Check sheet for the drawn part. Datum: minimum x, y, z corner. Units: mm. A direction names the side the tool comes from. Round coordinates to 2 decimals unless told otherwise and drop trailing zeros. Order: outer loops, then holes, each group sorted by start corner. A loop starts at its lowest first (then second) coordinate and runs counter-clockwise, first axis right, second up. Notation, with made-up numbers: (37.5, 68) -> (68.5, 68) arc R25 ccw to (68.5, 91) -> close; hole circle Ø6 at (-14.5, 69). An arc over 180 degrees is marked (long way). Answer in a Markdown table with one row per item.
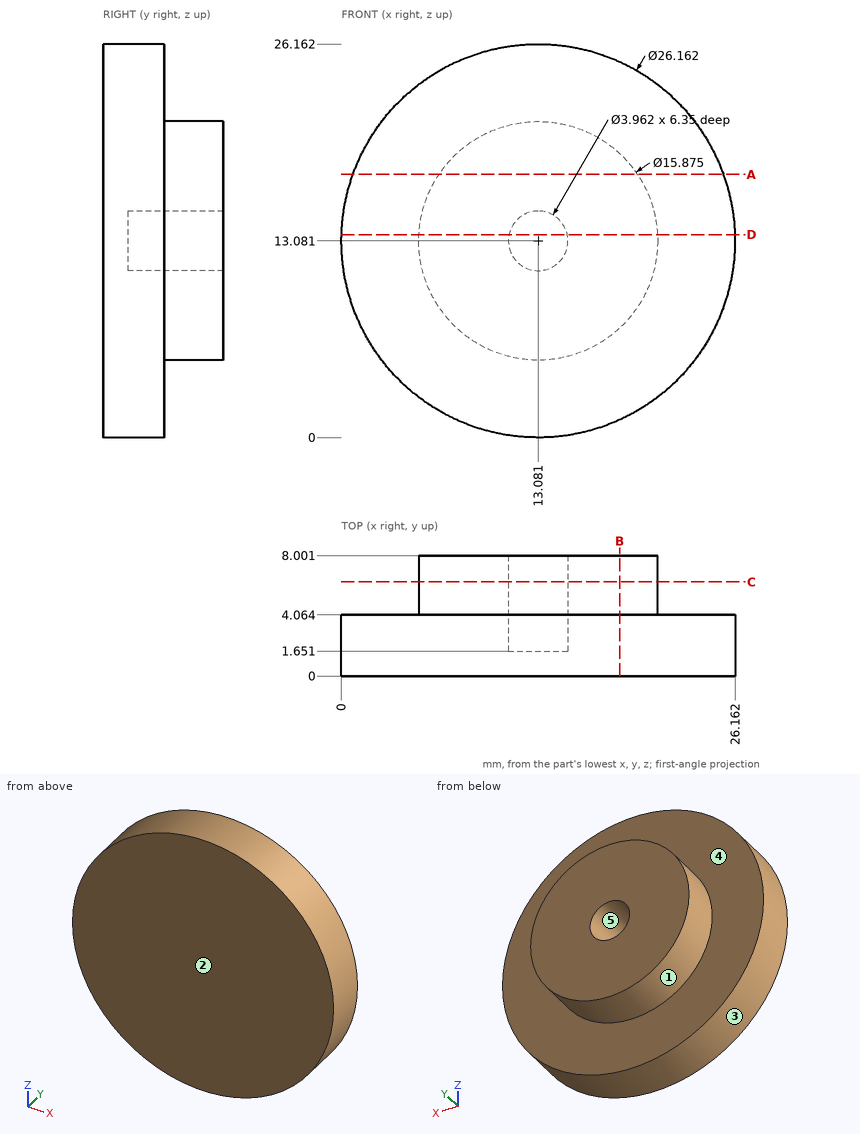
(1) Depth check by flat-ended pin: pin 1 Ø4 at (y, z) = (1.5, 21.5) entering from -X; pin 2 Ø1.2 at (x, z) = (12.5, 13) entering from +Y; pin 3 Ø2 at (y, z) = (6.5, 12) entering from +X. Enter the tip coordinate at first touch or a pass-through.
Solutions:
| item | result |
|---|---|
| pin 1 | x = 1.68 |
| pin 2 | y = 1.65 |
| pin 3 | x = 21.02 |
(2) Tool access check on the marked faces 1 and 2. Record the directions out of +Z, -Z, +X, -X, +Y, -Y that give a thin tool (end or side, any length) a straight path to the whole face; none if there is none.
Solutions:
| item | result |
|---|---|
| face 1 | +Y |
| face 2 | +Z, -Z, +X, -X, -Y |
(3) Section check B-B on x = 18.5. Record the boundary of the cut face in (y, z) (1 decimal), plus the area to 3 significant figures.
Solutions:
| item | result |
|---|---|
| outline | (0, 1.2) -> (4.1, 1.2) -> (4.1, 7.3) -> (8, 7.3) -> (8, 18.9) -> (4.1, 18.9) -> (4.1, 25) -> (0, 25) -> close |
| area | 142 mm^2 |
(4) Section check D-D on z = 13.5. Record the boundary of the cut face in (x, y) (1 decimal), plus the area to 3 significant figures.
Solutions:
| item | result |
|---|---|
| outline | (0, 0) -> (26.2, 0) -> (26.2, 4.1) -> (21, 4.1) -> (21, 8) -> (15, 8) -> (15, 1.7) -> (11.1, 1.7) -> (11.1, 8) -> (5.2, 8) -> (5.2, 4.1) -> (0, 4.1) -> close |
| area | 144 mm^2 |
(5) Section check A-A on z = 17.5. Record the boundary of the cut face in (x, y) (1 decimal), plus the area to 3 significant figures.
Solutions:
| item | result |
|---|---|
| outline | (0.8, 0) -> (25.4, 0) -> (25.4, 4.1) -> (19.7, 4.1) -> (19.7, 8) -> (6.5, 8) -> (6.5, 4.1) -> (0.8, 4.1) -> close |
| area | 152 mm^2 |
(6) Section check C-C on y = 6.25. Record the boundary of the cut face in (x, z) (1 decimal), plus the area to 3 significant figures.
Solutions:
| item | result |
|---|---|
| outline | circle Ø15.9 at (13.1, 13.1); hole circle Ø4 at (13.1, 13.1) |
| area | 186 mm^2 |
(7) Draft check along Z on the marked faces 3, 4 and 5. Enter one of: pulls with the +Z half, pulls with the -Z half, needs draft (parallel to the pull), parting line crosses it, or undercut.
Solutions:
| item | result |
|---|---|
| face 3 | parting line crosses it |
| face 4 | needs draft |
| face 5 | undercut |
(8) Scan lines: probe 1 along Y at (x, z) = (16, 22); probe 2 along X at (y, z) = (6, 12.5) (1 decimal); probe 3 along Z at (x, y) = (13.75, 2.5) (1 decimal). Record each from-to range of solid material in increasing order. Write a range as from..to.
Solutions:
| item | result |
|---|---|
| probe 1 | 0..4.06 |
| probe 2 | 5.2..11.2, 15..21 |
| probe 3 | 0..11.2, 14.9..26.1 |
